```python
from build123d import *

# Parameters (mm, degrees)
SKETCH1_R           = 2
SKETCH1_W           = 20
SKETCH1_H           = 50
SKETCH1_W_2         = 3.5
SKETCH1_H_2         = 22
SKETCH1_W_3         = 18
BOSS_EXTRUDE1_DEPTH = 2


with BuildPart() as part:
    # Sketch1 → Boss-Extrude1 (new body)
    with BuildSketch(Plane.XY):
        Polygon((0, -100), (-25, -96), (-30, -90), (-30, 90), (-25, 96), (0, 100), (25, 96), (30, 90), (30, -90), (25, -96), align=None)
        with Locations((-18, -91.5)):
            Circle(SKETCH1_R, mode=Mode.SUBTRACT)
        with Locations((-25, -30)):
            Circle(SKETCH1_R, mode=Mode.SUBTRACT)
        with Locations((-17.5, -18)):
            Circle(SKETCH1_R, mode=Mode.SUBTRACT)
        with Locations((0, -67)):
            Circle(SKETCH1_R, mode=Mode.SUBTRACT)
        with Locations((17.5, -18)):
            Circle(SKETCH1_R, mode=Mode.SUBTRACT)
        with Locations((25, -30)):
            Circle(SKETCH1_R, mode=Mode.SUBTRACT)
        with Locations((18, -91.5)):
            Circle(SKETCH1_R, mode=Mode.SUBTRACT)
        with Locations((18, 91.5)):
            Circle(SKETCH1_R, mode=Mode.SUBTRACT)
        with Locations((25, 30)):
            Circle(SKETCH1_R, mode=Mode.SUBTRACT)
        with Locations((17.5, 18)):
            Circle(SKETCH1_R, mode=Mode.SUBTRACT)
        with Locations((0, 67)):
            Circle(SKETCH1_R, mode=Mode.SUBTRACT)
        with Locations((-17.5, 18)):
            Circle(SKETCH1_R, mode=Mode.SUBTRACT)
        with Locations((-25, 30)):
            Circle(SKETCH1_R, mode=Mode.SUBTRACT)
        with Locations((-18, 91.5)):
            Circle(SKETCH1_R, mode=Mode.SUBTRACT)
        Rectangle(SKETCH1_W, SKETCH1_H, mode=Mode.SUBTRACT)
        with Locations((-20.75, -49)):
            Rectangle(SKETCH1_W_2, SKETCH1_H_2, mode=Mode.SUBTRACT)
        with Locations((0, -50)):
            Rectangle(SKETCH1_W_3, SKETCH1_H_2, mode=Mode.SUBTRACT)
        with Locations((-20.75, 0)):
            Rectangle(SKETCH1_W_2, SKETCH1_H_2, mode=Mode.SUBTRACT)
        with Locations((20.75, 0)):
            Rectangle(SKETCH1_W_2, SKETCH1_H_2, mode=Mode.SUBTRACT)
        with Locations((20.75, -49)):
            Rectangle(SKETCH1_W_2, SKETCH1_H_2, mode=Mode.SUBTRACT)
        with Locations((20.75, 49)):
            Rectangle(SKETCH1_W_2, SKETCH1_H_2, mode=Mode.SUBTRACT)
        with Locations((0, 50)):
            Rectangle(SKETCH1_W_3, SKETCH1_H_2, mode=Mode.SUBTRACT)
        with Locations((-20.75, 49)):
            Rectangle(SKETCH1_W_2, SKETCH1_H_2, mode=Mode.SUBTRACT)
    extrude(amount=BOSS_EXTRUDE1_DEPTH)


solid = part.part
```
CAD build for the part. Positions are in the model's coordinates, mm. Round coordinates to 2 decimals unless told otherwise and drop trailing zeros. Order: outer loops, then holes, each group sorted by start corner. A loop starts at its lowest first (then second) coordinate and runs counter-clockwise, first axis right, second up. Notation, with made-up numbers: (70, -8.5) -> (83, -8.5) arc R13 ccw to (83, -2.5) -> close; hole circle Ø1 at (10, 52). An arc over 180 degrees is marked (long way). Write item = value, one per line.
(1) Cut at D-D (z = 1.65). State how many separate pieces and enclosed holes the cut face has, plus the area to 3 significant figures.
Answers follow:
separate_pieces = 1
enclosed_holes = 23
area = 9,230 mm²
(2) Pull direction Y, two halves, no side cores. Call faces 1 (the flat face through (14, 1, 2)), 2 (the cylindrical face through (25, 28, 1)), 3 (the flat face through (27.5, -93, 1)), 4 (the flat face through (27.5, 93, 1)): +Y half, -Y half, draft (parallel to the pull), parting line (faces both ways), or undercut.
Answers follow:
face_1 = draft
face_2 = undercut
face_3 = -Y half
face_4 = +Y half
(3) Cut at B-B (y = 30). Write the cut outline in (x, z), plus the area to 3 significant figures.
Answers follow:
outline = (-30, 0) -> (-27, 0) -> (-27, 2) -> (-30, 2) -> close; (-23, 0) -> (23, 0) -> (23, 2) -> (-23, 2) -> close; (27, 0) -> (30, 0) -> (30, 2) -> (27, 2) -> close
area = 104 mm²
(4) Cut at A-A (x = 5.5). Write the cut outline in (y, z).
Answers follow:
outline = (-99.12, 0) -> (-61, 0) -> (-61, 2) -> (-99.12, 2) -> close; (-39, 0) -> (-25, 0) -> (-25, 2) -> (-39, 2) -> close; (25, 0) -> (39, 0) -> (39, 2) -> (25, 2) -> close; (61, 0) -> (99.12, 0) -> (99.12, 2) -> (61, 2) -> close
(5) Flat gauge pins, fed straight in: P1, Ø0.6, axis at x = -20, z = 1, coming from the +Y side; P2, Ø2.5, axis at x = 18, y = 91.5, coming from the +Z side; P3, Ø0.6, axis at x = 21, z = 1, coming from the -Y side. Where does each tip first touch, or does it go through?
Answers follow:
P1 = 96.85
P2 = through
P3 = -96.69
(6) Drill centre lines: L1, parallel to X at y = -59, z = 1.25; L2, parallel to Y at x = -25, z = 1.2; L3, parallel to X at y = 5, z = 0.35. Where is each one in solid material? Low to high.
Answers follow:
L1 = -30 to -22.5, -19 to -9, 9 to 19, 22.5 to 30
L2 = -96 to -32, -28 to 28, 32 to 96
L3 = -30 to -22.5, -19 to -10, 10 to 19, 22.5 to 30
(7) Cut at C-C (y = -67). Write the cut outline in (x, z).
Answers follow:
outline = (-30, 0) -> (-2, 0) -> (-2, 2) -> (-30, 2) -> close; (2, 0) -> (30, 0) -> (30, 2) -> (2, 2) -> close
